Part model, mm, in its own coordinate system. Face numbers are marked on the shaded views. A direction names the side the tool comes from. Round coordinates to 2 decimals unless told otherwise and drop trailing zeros. Loops run counter-clockwise (first coordinate to the right, second up) from the corner with the lowest first, then second, coordinate; pieces in that order, holes last. Notation, with made-up numbers: (-11, -30.75) - (26, -30.75) arc R27 cw to (26, -0.75) - close; hole circle Ø10 at (-1.75, -5). An arc over 180 degrees is marked (long way). Write each question's results on one line, items separated by ' | '. Start each with the question number.
(1) Cut at A-A, the plane y = 0. List the corners of the cut face in (x, z), then the cut area to 4 significant figures.
(2) Cut at C-C, the plane x = 32.5. List the corners of the cut face in (y, z).
(3) Drill centre lines: L1, parallel to Y at x = -26.5, z = 36; L2, parallel to Y at x = 26.5, z = 33; L3, parallel to Y at x = 0, z = 36.9. Where is each one in solid material? Low to high.
(4) Cut at B-B, the plane x = 0. List the corners of the cut face in (y, z).
(5) Flat gauge pin, fed straight in: P1, Ø12, axis at y = -0.5, z = 34, coming from the -X side. Where does the tip first touch, or does it go through?
(6) Tool access for the marked faces 4 and 5: list every direction of +Z, -Z, +X, -X, +Y, -Y with a clear straight run to the whole face (end or side of a thin tool).
(7) Mould opens along X. For the marked faces 1, 2 and 3 say: released by +X, released by -X, zero draft, split by the parting line, or undercut.
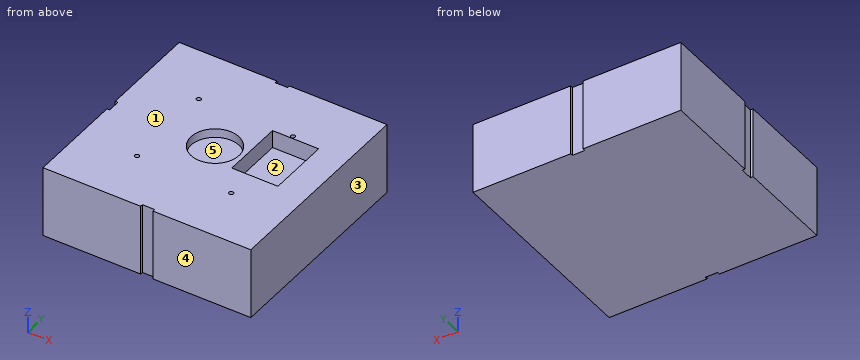
from build123d import *

# Parameters (mm, degrees)
SKETCH1_W            = 117
SKETCH1_H            = 117
BODY_DEPTH           = 40
SKETCH4_W            = 7
SKETCH4_H            = 3
SKETCH4_W_2          = 3
SKETCH4_H_2          = 7
RAILS_HOUSINGS_DEPTH = 41
DRILL_START          = -40
SKETCH6_R            = 1.25
DRILL_HOLES_DEPTH    = 10
PCB_START            = -40
SKETCH7_W            = 26
SKETCH7_H            = 35
PCB_GAP_DEPTH        = 10
MOTOR_START          = -40
SKETCH8_R            = 13.5
MOTOR_GAP_DEPTH      = 5
SKETCH13_W           = 40
SKETCH13_H           = 7
BOSS_EXTRUDE4_DEPTH  = 1.5


with BuildPart() as part:
    # Sketch1 → body (new body)
    with BuildSketch(Plane.XY):
        Rectangle(SKETCH1_W, SKETCH1_H)
    extrude(amount=BODY_DEPTH)

    # Sketch4 → rails housings (cut, through all)
    with BuildSketch(Plane(origin=(0, 0, 0), x_dir=(-1, 0, 0), z_dir=(0, 0, -1))):
        with Locations((0, 58.5)):
            Rectangle(SKETCH4_W, SKETCH4_H)
        with Locations((58.5, 0)):
            Rectangle(SKETCH4_W_2, SKETCH4_H_2)
        with Locations((0, -58.5)):
            Rectangle(SKETCH4_W, SKETCH4_H)
        with Locations((-58.5, 0)):
            Rectangle(SKETCH4_W_2, SKETCH4_H_2)
    extrude(amount=-RAILS_HOUSINGS_DEPTH, mode=Mode.SUBTRACT)

    # Sketch6 → drill holes (cut)
    with BuildSketch(Plane(origin=(0, 0, 0), x_dir=(-1, 0, 0), z_dir=(0, 0, -1)).offset(DRILL_START)):
        with Locations((-26.5, 26.5)):
            Circle(SKETCH6_R)
        with Locations((26.5, 26.5)):
            Circle(SKETCH6_R)
        with Locations((26.5, -26.5)):
            Circle(SKETCH6_R)
        with Locations((-26.5, -26.5)):
            Circle(SKETCH6_R)
    extrude(amount=DRILL_HOLES_DEPTH, mode=Mode.SUBTRACT)

    # Sketch7 → PCB gap (cut)
    with BuildSketch(Plane(origin=(0, 0, 0), x_dir=(-1, 0, 0), z_dir=(0, 0, -1)).offset(PCB_START)):
        with Locations((-29, 7.5)):
            Rectangle(SKETCH7_W, SKETCH7_H)
    extrude(amount=PCB_GAP_DEPTH, mode=Mode.SUBTRACT)

    # Sketch8 → motor gap (cut)
    with BuildSketch(Plane(origin=(0, 0, 0), x_dir=(-1, 0, 0), z_dir=(0, 0, -1)).offset(MOTOR_START)):
        Circle(SKETCH8_R)
    extrude(amount=MOTOR_GAP_DEPTH, mode=Mode.SUBTRACT)

    # Sketch13 → Boss-Extrude4 (add)
    with BuildSketch(Plane(origin=(57, 0, 0), x_dir=(0, 0, -1), z_dir=(1, 0, 0))):
        with Locations((-20, 0)):
            Rectangle(SKETCH13_W, SKETCH13_H)
    extrude(amount=BOSS_EXTRUDE4_DEPTH)


solid = part.part
A:
1) outline: (-57, 0) - (58.5, 0) - (58.5, 40) - (42, 40) - (42, 30) - (16, 30) - (16, 40) - (13.5, 40) - (13.5, 35) - (-13.5, 35) - (-13.5, 40) - (-57, 40) - close | area: 4,225 mm2
2) outline: (-58.5, 0) - (58.5, 0) - (58.5, 40) - (25, 40) - (25, 30) - (-10, 30) - (-10, 40) - (-58.5, 40) - close
3) L1: -58.5 to -27.75, -25.25 to 25.25, 27.75 to 58.5 | L2: -58.5 to -27.75, -25.25 to -10, 25 to 25.25, 27.75 to 58.5 | L3: -57 to -13.5, 13.5 to 57
4) outline: (-57, 0) - (57, 0) - (57, 40) - (13.5, 40) - (13.5, 35) - (-13.5, 35) - (-13.5, 40) - (-57, 40) - close
5) P1: x = -58.5
6) face 4: +Z, -Z, +X, -X, -Y | face 5: +Z
7) face 1: zero draft | face 2: undercut | face 3: released by +X
